For this review, take the finished solid that the model builds, in its own axes (mm). Face numbers are marked on the shaded views. A direction names the side the tool comes from. Coordinates: 2 decimals unless noted, no trailing zeros. Write each loop counter-clockwise with the first axis right and the second up, starting at its lowest first coordinate (ties: lowest second). Pieces come first, ordered by that corner, then holes. Notation, with made-up numbers: M 67.5,64 L 112.5,64 A19 ccw 112.5,70 Z; hole C 24,10.5 d1. An arc over 180 degrees is marked long. Return JSON: item names as keys, results as strings.
```python
from build123d import *

# Parameters (mm, degrees)
BOSS_EXTRUDE1_DEPTH      = 4.3
BOSS_EXTRUDE1_DEPTH_BACK = 4
SKETCH1_R                = 4.65
SKETCH2_R                = 2.35
BOSS_EXTRUDE2_DEPTH      = 20.68
CUT_EXTRUDE1_START       = -4
SKETCH3_R                = 2.35
SKETCH3_R_2              = 1.85
CUT_EXTRUDE1_DEPTH       = 2
CUT_EXTRUDE2_START       = -2
SKETCH4_R                = 4.65
SKETCH4_R_2              = 2.65
CUT_EXTRUDE2_DEPTH       = 1.5
FILLET1_R                = 1


with BuildPart() as part:
    # Sketch1 → Boss-Extrude1 (new, two sides: drawn at the far end of the back side and taken through both)
    with BuildSketch(Plane(origin=(0, 0, 0), x_dir=(1, 0, 0), z_dir=(0, 1, 0)).offset(-BOSS_EXTRUDE1_DEPTH_BACK)):
        with Locations(Location((0, 0, 0), (0, 0, 270))):
            Circle(SKETCH1_R)
    extrude(amount=BOSS_EXTRUDE1_DEPTH + BOSS_EXTRUDE1_DEPTH_BACK)

    # Sketch2 → Boss-Extrude2 (add)
    with BuildSketch(Plane(origin=(0, 4.3, 0), x_dir=(1, 0, 0), z_dir=(0, 1, 0))):
        with Locations(Location((0, 0, 0), (0, 0, 270))):
            Circle(SKETCH2_R)
    extrude(amount=BOSS_EXTRUDE2_DEPTH)

    # Sketch3 → Cut-Extrude1 (cut)
    with BuildSketch(Plane(origin=(0, 24.98, 0), x_dir=(1, 0, 0), z_dir=(0, 1, 0)).offset(CUT_EXTRUDE1_START)):
        with Locations(Location((0, 0, 0), (0, 0, 270))):
            Circle(SKETCH3_R)
        with Locations(Location((0, 0, 0), (0, 0, 270))):
            Circle(SKETCH3_R_2, mode=Mode.SUBTRACT)
    extrude(amount=CUT_EXTRUDE1_DEPTH, mode=Mode.SUBTRACT)

    # Sketch4 → Cut-Extrude2 (cut)
    with BuildSketch(Plane.XZ.offset(4).offset(CUT_EXTRUDE2_START)):
        with Locations(Location((0, 0, 0), (0, 0, 90))):
            Circle(SKETCH4_R)
        with Locations(Location((0, 0, 0), (0, 0, 270))):
            Circle(SKETCH4_R_2, mode=Mode.SUBTRACT)
    extrude(amount=-CUT_EXTRUDE2_DEPTH, mode=Mode.SUBTRACT)

    # Fillet1
    # the kernel refuses this fillet: 1 mm, written as the material it adds along each edge
    with BuildSketch(Plane(origin=(0, 20.98, 0), x_dir=(0, 0, 1), z_dir=(-1, 0, 0))) as fillet1_piece_1:
        with BuildLine():
            CenterArc((2.85, 0.866025404), FILLET1_R, 180, 60)
            Line((1.85, 0.866025404), (1.83, 0.866025404))
            Line((1.83, 0.866025404), (1.83, 0))
            Line((1.83, 0), (1.85, -0.02))
            ThreePointArc((1.85, -0.02), (2.1, -0.02), (2.34, -0.017320508))
            Line((2.34, -0.017320508), (2.35, 0))
        make_face()
    revolve(axis=Axis((0, 20.98, 0), (0, 1, 0)))
    with BuildSketch(Plane(origin=(0, 22.98, 0), x_dir=(0, 0, 1), z_dir=(-1, 0, 0))) as fillet1_piece_2:
        with BuildLine():
            CenterArc((2.85, -0.866025404), FILLET1_R, 120, 60)
            Line((2.35, 0), (2.34, 0.017320508))
            ThreePointArc((2.34, 0.017320508), (2.1, 0.02), (1.85, 0.02))
            Line((1.85, 0.02), (1.83, 0))
            Line((1.83, 0), (1.83, -0.866025404))
            Line((1.83, -0.866025404), (1.85, -0.866025404))
        make_face()
    revolve(axis=Axis((0, 22.98, 0), (0, 1, 0)))


solid = part.part
```
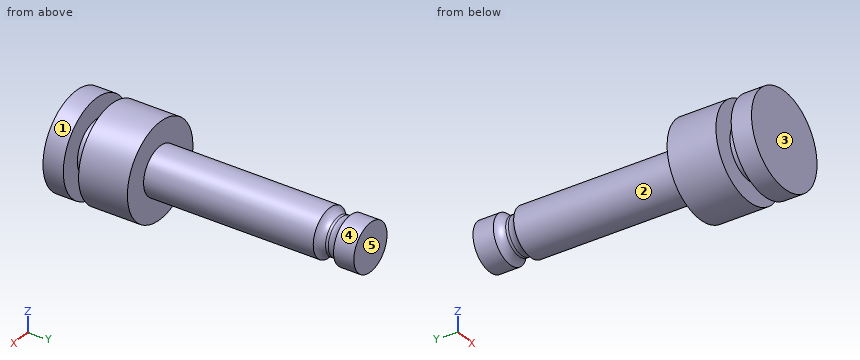
1. Wall thickness on L1, parallel to Y at x = 0.75, z = 3.25; L2, parallel to Y at x = 0.25, z = 2.5; L3, parallel to Z at x = -1.75, y = 18: over which ranges is each line inside the solid? List them lowest first. Write a range as from..to.
Checks:
{"L1": "-4..-2, -0.5..4.3", "L2": "-4..4.3", "L3": "-1.57..1.57"}
2. We need section B-B (x = 4.25). State the section outline as (y, z) points.
Checks:
{"outline": "M -4,-1.89 L -2,-1.89 L -2,1.89 L -4,1.89 Z; M -0.5,-1.89 L 4.3,-1.89 L 4.3,1.89 L -0.5,1.89 Z"}
3. Clearance check with flat-ended pins moving along their axes: pin 1 Ø1 at (y, z) = (20, -3) entering from -X; pin 2 Ø5 at (y, z) = (15, -3) entering from +X; pin 3 Ø2 at (x, y) = (0, 5.5) entering from +Z; pin 4 Ø2 at (x, y) = (-1.5, 11) entering from -Z. State where each tip first meets the part, or that it passes through.
Checks:
{"pin 1": "through", "pin 2": "x = 2.3", "pin 3": "z = 2.35", "pin 4": "z = -2.3"}
4. Draft analysis for pull direction Y (two halves, no side actions). For the marked faces 3, 4 and 5, state which applies: +Y half, -Y half, draft (parallel to the pull), parting line (faces both ways), or undercut.
Checks:
{"face 3": "-Y half", "face 4": "draft", "face 5": "+Y half"}
5. We need section D-D (z = 0). State the section outline as (x, y) points, plus the area to 3 significant figures.
Checks:
{"outline": "M -4.65,-4 L 4.65,-4 L 4.65,-2 L 2.65,-2 L 2.65,-0.5 L 4.65,-0.5 L 4.65,4.3 L 2.35,4.3 L 2.35,20.98 A1 cw 1.85,21.85 L 1.85,22.11 A1 cw 2.35,22.98 L 2.35,24.98 L -2.35,24.98 L -2.35,22.98 A1 cw -1.85,22.11 L -1.85,21.85 A1 cw -2.35,20.98 L -2.35,4.3 L -4.65,4.3 L -4.65,-0.5 L -2.65,-0.5 L -2.65,-2 L -4.65,-2 Z", "area": "167 mm2"}
6. For the marked faces 1 and 2, list the 3-axis set-ups (+Z, -Z, +X, -X, +Y, -Y) from which the entire face can be reached by the end or side of a thin tool; tool diameter is ignored.
Checks:
{"face 1": "+Y, -Y", "face 2": "+Y"}
7. We need section C-C (x = 0). State the section outline as (y, z) points.
Checks:
{"outline": "M -4,-4.65 L -2,-4.65 L -2,-2.65 L -0.5,-2.65 L -0.5,-4.65 L 4.3,-4.65 L 4.3,-2.35 L 20.98,-2.35 A1 cw 21.85,-1.85 L 22.11,-1.85 A1 cw 22.98,-2.35 L 24.98,-2.35 L 24.98,2.35 L 22.98,2.35 A1 cw 22.11,1.85 L 21.85,1.85 A1 cw 20.98,2.35 L 4.3,2.35 L 4.3,4.65 L -0.5,4.65 L -0.5,2.65 L -2,2.65 L -2,4.65 L -4,4.65 Z"}
8. We need section A-A (z = -3.5). State the section outline as (x, y) points.
Checks:
{"outline": "M -3.06,-4 L 3.06,-4 L 3.06,-2 L -3.06,-2 Z; M -3.06,-0.5 L 3.06,-0.5 L 3.06,4.3 L -3.06,4.3 Z"}
